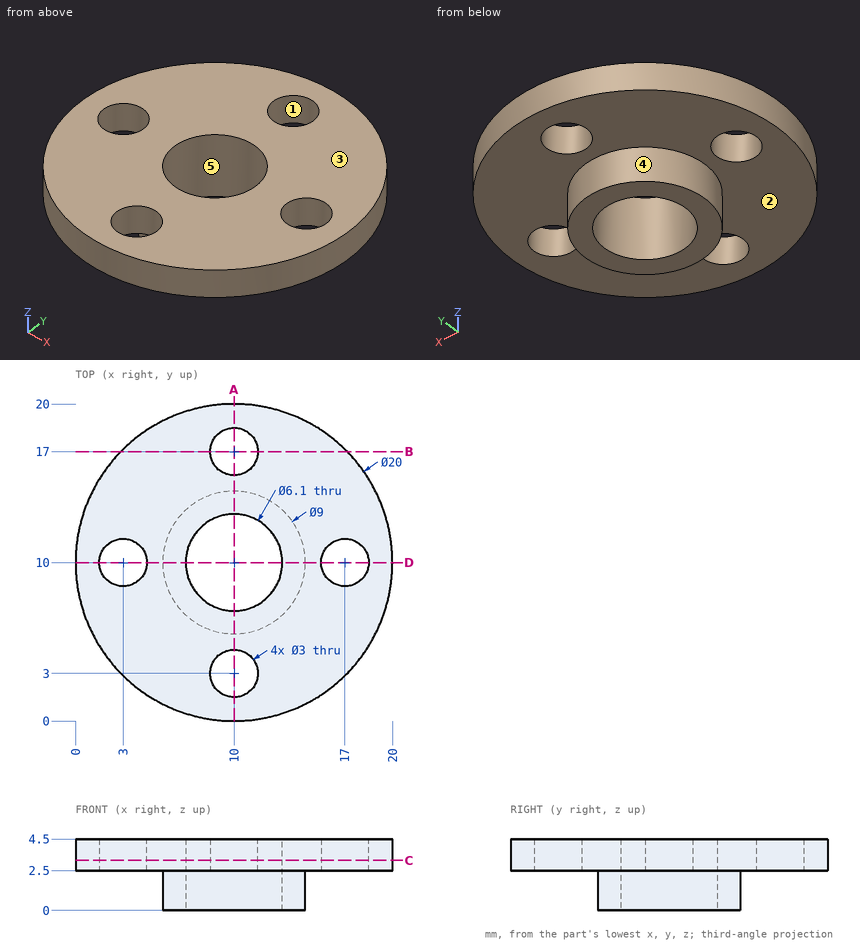
Print and shaded views of the part. All mm, measured from the part's lowest x, y and z. A direction names the side the tool comes from. Round coordinates to 2 decimals unless told otherwise and drop trailing zeros. Order: outer loops, then holes, each group sorted by start corner. A loop starts at its lowest first (then second) coordinate and runs counter-clockwise, first axis right, second up.
Q1. Slice it at C-C (z = 3.15). Write the cut outline in (x, y), and give its area (3 significant figures).
Q2. Slice it at A-A (x = 10). Write the cut outline in (y, z), and give its area (4 significant figures).
Q3. Wall check: L1, parallel to Y at x = 10, z = 3.05; L2, parallel to X at y = 8.75, z = 3; L3, parallel to X at y = 9.5, z = 3.55. Give the ranges that are in metal, low to high.
Q4. Two-plate mould, pull along X, no slides. Class the marked faces 3, 4 and 5: pulls with the +X half, pulls with the -X half, needs draft (parallel to the pull), parting line crosses it, or undercut.
Q5. Drop flat-ended pins along their axis: pin 1 (2.5 mm diameter, centred on x = 10, y = 17, fed in from -Z); pin 2 (2 mm diameter, centred on x = 13, y = 16.5, fed in from -Z); pin 3 (1 mm diameter, centred on y = 10, z = 0.5, fed in from -X); pin 4 (2 mm diameter, centred on x = 11.5, z = 4, fed in from -Y). Give the stop position or say it passes through.
Q6. Slice it at B-B (y = 17). Write the cut outline in (x, z), and give its area (3 significant figures).
Q7. Which spindle directions (+Z, -Z, +X, -X, +Y, -Y) get a long thin tool onto all of the face, cutting with end or side? Do the marked faces 1 and 2. Say none if no direction does.
Results below:
1. outline: circle Ø20 at (10, 10); hole circle Ø3 at (3, 10); hole circle Ø6.1 at (10, 10); hole circle Ø3 at (10, 3); hole circle Ø3 at (10, 17); hole circle Ø3 at (17, 10)
1. area: 257 mm2
2. outline: (0, 2.5) - (1.5, 2.5) - (1.5, 4.5) - (0, 4.5) - close; (4.5, 2.5) - (5.5, 2.5) - (5.5, 0) - (6.95, 0) - (6.95, 4.5) - (4.5, 4.5) - close; (13.05, 0) - (14.5, 0) - (14.5, 2.5) - (15.5, 2.5) - (15.5, 4.5) - (13.05, 4.5) - close; (18.5, 2.5) - (20, 2.5) - (20, 4.5) - (18.5, 4.5) - close
2. area: 23.05 mm2
3. L1: y = 0 to 1.5, 4.5 to 6.95, 13.05 to 15.5, 18.5 to 20
3. L2: x = 0.08 to 2.17, 3.83 to 7.22, 12.78 to 16.17, 17.83 to 19.92
3. L3: x = 0.01 to 1.59, 4.41 to 6.99, 13.01 to 15.59, 18.41 to 19.99
4. face 3: needs draft
4. face 4: parting line crosses it
4. face 5: undercut
5. pin 1: passes through
5. pin 2: stops at z = 2.5
5. pin 3: stops at x = 5.5
5. pin 4: stops at y = 0.01
6. outline: (2.86, 2.5) - (8.5, 2.5) - (8.5, 4.5) - (2.86, 4.5) - close; (11.5, 2.5) - (17.14, 2.5) - (17.14, 4.5) - (11.5, 4.5) - close
6. area: 22.6 mm2
7. face 1: +Z, -Z
7. face 2: -Z
